```python
from build123d import *

# Parameters (mm, degrees)
SKETCH1_W                    = 110
SKETCH1_H                    = 200
SKETCH1_W_2                  = 70
SKETCH1_H_2                  = 120
BASE_FLANGE1_DEPTH           = 0.7366
EDGE_FLANGE1_STRIP_W         = 4.4196
EDGE_FLANGE1_STRIP_H         = 0.7366
EDGE_FLANGE1_STRIP_CUT_DEPTH = 200
EDGE_FLANGE1_DEPTH           = 200
EDGE_FLANGE2_STRIP_W         = 4.4196
EDGE_FLANGE2_STRIP_H         = 0.7366
EDGE_FLANGE2_STRIP_CUT_DEPTH = 200
EDGE_FLANGE2_DEPTH           = 200
EDGE_FLANGE3_STRIP_W         = 4.4196
EDGE_FLANGE3_STRIP_H         = 0.7366
EDGE_FLANGE3_STRIP_CUT_DEPTH = 108.5268
EDGE_FLANGE3_DEPTH           = 108.5268
EDGE_FLANGE3_START           = 0.7366
EDGE_FLANGE3_FLAT_DEPTH      = 0.7366
EDGE_FLANGE4_STRIP_W         = 4.4196
EDGE_FLANGE4_STRIP_H         = 0.7366
EDGE_FLANGE4_STRIP_CUT_DEPTH = 108.5268
EDGE_FLANGE4_DEPTH           = 108.5268
EDGE_FLANGE4_START           = 0.7366
EDGE_FLANGE4_FLAT_DEPTH      = 0.7366
CUT_EXTRUDE2_DEPTH           = 289.797370967
CUT_EXTRUDE3_START           = -0.7366
CUT_EXTRUDE3_DEPTH           = 0.7366
CUT_EXTRUDE6_DEPTH           = 800.082459726
CUT_EXTRUDE6_DEPTH_BACK      = 800.082459726
SKETCH53_R                   = 2.2
SKETCH53_R_2                 = 2.199999998
CUT_EXTRUDE7_DEPTH           = 10


# Read off the part's stored shape, not the designer's step: Cut-Extrude3
# Sheet-metal steps are written as plain solids
with BuildPart() as part:
    # Sketch1 → Base-Flange1 (new body)
    with BuildSketch(Plane(origin=(0, 0, 0), x_dir=(1, 0, 0), z_dir=(0, 1, 0))):
        Rectangle(SKETCH1_W, SKETCH1_H)
        Rectangle(SKETCH1_W_2, SKETCH1_H_2, mode=Mode.SUBTRACT)
    extrude(amount=-BASE_FLANGE1_DEPTH)

    # Edge-Flange1 strip (across the edge) → Edge-Flange1 strip cut (cut)
    with BuildSketch(Plane(origin=(-55, 0, -100), x_dir=(1, 0, 0), z_dir=(0, 0, 1))):
        with Locations((-1.4732, -0.3683)):
            Rectangle(EDGE_FLANGE1_STRIP_W, EDGE_FLANGE1_STRIP_H)
    extrude(amount=EDGE_FLANGE1_STRIP_CUT_DEPTH, mode=Mode.SUBTRACT)

    # Edge-Flange1 section (across the edge) → Edge-Flange1 (add)
    with BuildSketch(Plane(origin=(-55, 0, -100), x_dir=(1, 0, 0), z_dir=(0, 0, 1))):
        with BuildLine():
            Line((-0.7366, 0.7366), (-0.7366, 199.2634))
            Line((-0.7366, 199.2634), (0, 199.2634))
            Line((0, 199.2634), (0, 0.7366))
            ThreePointArc((0, 0.7366), (0.215745145, 0.215745145), (0.7366, 0))
            Line((0.7366, 0), (0.7366, -0.7366))
            ThreePointArc((0.7366, -0.7366), (-0.30510971, -0.30510971), (-0.7366, 0.7366))
        make_face()
    extrude(amount=EDGE_FLANGE1_DEPTH)

    # Edge-Flange2 strip (across the edge) → Edge-Flange2 strip cut (cut)
    with BuildSketch(Plane(origin=(55, 0, 100), x_dir=(-1, 0, 0), z_dir=(0, 0, -1))):
        with Locations((-1.4732, -0.3683)):
            Rectangle(EDGE_FLANGE2_STRIP_W, EDGE_FLANGE2_STRIP_H)
    extrude(amount=EDGE_FLANGE2_STRIP_CUT_DEPTH, mode=Mode.SUBTRACT)

    # Edge-Flange2 section (across the edge) → Edge-Flange2 (add)
    with BuildSketch(Plane(origin=(55, 0, 100), x_dir=(-1, 0, 0), z_dir=(0, 0, -1))):
        with BuildLine():
            Line((-0.7366, 0.7366), (-0.7366, 99.2634))
            Line((-0.7366, 99.2634), (0, 99.2634))
            Line((0, 99.2634), (0, 0.7366))
            ThreePointArc((0, 0.7366), (0.215745145, 0.215745145), (0.7366, 0))
            Line((0.7366, 0), (0.7366, -0.7366))
            ThreePointArc((0.7366, -0.7366), (-0.30510971, -0.30510971), (-0.7366, 0.7366))
        make_face()
    extrude(amount=EDGE_FLANGE2_DEPTH)

    # Edge-Flange3 strip (across the edge) → Edge-Flange3 strip cut (cut)
    with BuildSketch(Plane(origin=(54.2634, 0, -100), x_dir=(0, 0, 1), z_dir=(-1, 0, 0))):
        with Locations((-1.4732, -0.3683)):
            Rectangle(EDGE_FLANGE3_STRIP_W, EDGE_FLANGE3_STRIP_H)
    extrude(amount=EDGE_FLANGE3_STRIP_CUT_DEPTH, mode=Mode.SUBTRACT)

    # Edge-Flange3 bend section (across the edge) → Edge-Flange3 (add)
    with BuildSketch(Plane(origin=(54.2634, 0, -100), x_dir=(0, 0, 1), z_dir=(-1, 0, 0))):
        with BuildLine():
            Line((-0.7366, 0.7366), (0, 0.7366))
            ThreePointArc((0, 0.7366), (0.215745145, 0.215745145), (0.7366, 0))
            Line((0.7366, 0), (0.7366, -0.7366))
            ThreePointArc((0.7366, -0.7366), (-0.30510971, -0.30510971), (-0.7366, 0.7366))
        make_face()
    extrude(amount=EDGE_FLANGE3_DEPTH)

    # Edge-Flange3 profile (on flange) → Edge-Flange3 flat (add)
    with BuildSketch(Plane(origin=(0, 0, -100), x_dir=(-1, 0, 0), z_dir=(0, 0, -1)).offset(EDGE_FLANGE3_START)):
        Polygon((-54.2634, 115), (-54.2634, 0.7366), (54.2634, 0.7366), (54.2634, 199.2634), align=None)
    extrude(amount=-EDGE_FLANGE3_FLAT_DEPTH)

    # Edge-Flange4 strip (across the edge) → Edge-Flange4 strip cut (cut)
    with BuildSketch(Plane(origin=(-54.2634, 0, 100), x_dir=(0, 0, -1), z_dir=(1, 0, 0))):
        with Locations((-1.4732, -0.3683)):
            Rectangle(EDGE_FLANGE4_STRIP_W, EDGE_FLANGE4_STRIP_H)
    extrude(amount=EDGE_FLANGE4_STRIP_CUT_DEPTH, mode=Mode.SUBTRACT)

    # Edge-Flange4 bend section (across the edge) → Edge-Flange4 (add)
    with BuildSketch(Plane(origin=(-54.2634, 0, 100), x_dir=(0, 0, -1), z_dir=(1, 0, 0))):
        with BuildLine():
            Line((-0.7366, 0.7366), (0, 0.7366))
            ThreePointArc((0, 0.7366), (0.215745145, 0.215745145), (0.7366, 0))
            Line((0.7366, 0), (0.7366, -0.7366))
            ThreePointArc((0.7366, -0.7366), (-0.30510971, -0.30510971), (-0.7366, 0.7366))
        make_face()
    extrude(amount=EDGE_FLANGE4_DEPTH)

    # Edge-Flange4 profile (on flange) → Edge-Flange4 flat (add)
    with BuildSketch(Plane.XY.offset(100).offset(EDGE_FLANGE4_START)):
        Polygon((-54.2634, 199.2634), (-54.2634, 0.7366), (54.2634, 0.7366), (54.2634, 115), align=None)
    extrude(amount=-EDGE_FLANGE4_FLAT_DEPTH)

    # Sketch24 → Cut-Extrude2 (cut, through all)
    with BuildSketch(Plane(origin=(0, 0, -100.7366), x_dir=(-1, 0, 0), z_dir=(0, 0, -1))):
        Polygon((-28.519875042, 107.808063094), (31.460124178, 107.808063094), (31.460124178, 158.533542729), align=None)
        Polygon((-28.150641863, 10.732953924), (31.829357358, 10.732953924), (31.829357358, 61.45843356), align=None)
        Polygon((31.713150602, 88.173102361), (-28.636081798, 88.173102361), (-28.636081798, 37.135359798), align=None)
    extrude(amount=-CUT_EXTRUDE2_DEPTH, mode=Mode.SUBTRACT)

    # Cut-Extrude3 outline → Cut-Extrude3 (cut)
    with BuildSketch(Plane(origin=(55.7366, 0, 0), x_dir=(0, 0, -1), z_dir=(1, 0, 0)).offset(CUT_EXTRUDE3_START)):
        with BuildLine():
            Line((-87.713422796, 42.053472661), (-6.797155753, 39.040000774))
            add(Edge.make_bspline(
                [(-6.797155753, 39.040000774), (-87.713422796, 42.053472661), (67.110125935, 80.068334048), (60.312641059, 39.424036929), (22.052524279, 39.424036929)],
                knots=[0, 0, 0, 0, 0, 1, 1, 1, 1, 1], degree=4))
            Line((22.052524279, 39.424036929), (60.312641059, 39.424036929))
            ThreePointArc((60.312641059, 39.424036929), (80.917037974, 56.86865569), (67.110125935, 80.068334048))
            Line((67.110125935, 80.068334048), (-87.713422796, 42.053472661))
        make_face()
    extrude(amount=CUT_EXTRUDE3_DEPTH, mode=Mode.SUBTRACT)

    # Sketch53 → Cut-Extrude6 (cut, two sides: drawn at the far end of the back side and taken through both)
    with BuildSketch(Plane(origin=(344.115063699, 0, 561.793038506), x_dir=(-1, 0, 0), z_dir=(0, 1, 0)).offset(-CUT_EXTRUDE6_DEPTH_BACK)):
        with Locations(Location((392.463649434, -480.956438506, 0), (0, 0, 90))):
            Circle(SKETCH53_R)
        with Locations(Location((392.463649434, -465.956438506, 0), (0, 0, 90))):
            Circle(SKETCH53_R)
        with Locations(Location((362.463649434, -473.456438506, 0), (0, 0, 90))):
            Circle(SKETCH53_R)
        with Locations(Location((292.463649434, -480.956438506, 0), (0, 0, 90))):
            Circle(SKETCH53_R)
        with Locations(Location((292.463649434, -465.956438506, 0), (0, 0, 90))):
            Circle(SKETCH53_R)
        with Locations(Location((322.463649434, -473.456438506, 0), (0, 0, 90))):
            Circle(SKETCH53_R)
        with Locations(Location((294.03158687, -636.983238506, 0), (0, 0, 90))):
            Circle(SKETCH53_R_2)
        with Locations(Location((324.69158687, -646.983238506, 0), (0, 0, 90))):
            Circle(SKETCH53_R_2)
        with Locations(Location((346.36158687, -636.983238506, 0), (0, 0, 90))):
            Circle(SKETCH53_R_2)
        with Locations(Location((368.028253537, -646.983238506, 0), (0, 0, 90))):
            Circle(SKETCH53_R_2)
        with Locations(Location((389.694920203, -636.983238506, 0), (0, 0, 90))):
            Circle(SKETCH53_R_2)
    extrude(amount=CUT_EXTRUDE6_DEPTH + CUT_EXTRUDE6_DEPTH_BACK, mode=Mode.SUBTRACT)

    # Sketch54 → Cut-Extrude7 (cut)
    with BuildSketch(Plane.ZY.offset(55.7366)):
        Polygon((-37.376001553, 179.2634), (5.247996894, 179.2634), (80, 105.199675962), (80, 62.968137981), align=None)
        Polygon((-80, 179.2634), (-80, 137.031862019), (37.376001553, 20.7366), (80, 20.7366), align=None)
        Polygon((-47.87199534, 20.7366), (-5.247996894, 20.7366), (-80, 94.800324038), (-80, 52.568786057), align=None)
        Polygon((80, 179.2634), (80, 147.431213943), (47.87199534, 179.2634), align=None)
    extrude(amount=-CUT_EXTRUDE7_DEPTH, mode=Mode.SUBTRACT)


solid = part.part
```
For this review, take the finished solid that the model builds, in its own axes (mm). A direction names the side the tool comes from. Coordinates: 2 decimals unless noted, no trailing zeros. Order: outer loops, then holes, each group sorted by start corner. A loop starts at its lowest first (then second) coordinate and runs counter-clockwise, first axis right, second up. Notation, with made-up numbers: (67.25, 60) -> (93.25, 60) arc R6 cw to (93.25, 65) -> close; hole circle Ø7 at (13.25, 21.25). An arc over 180 degrees is marked (long way). Answer as CSV lines item,"result".
Q1. We need section B-B (z = -70). State the section outline as (x, y) points.
Model answer:
outline,"(-55.74, 0.74) arc R1.47 ccw to (-54.26, -0.74) -> (54.26, -0.74) arc R1.47 ccw to (55.74, 0.74) -> (55.74, 41.81) -> (55, 41.81) -> (55, 0.74) arc R0.74 cw to (54.26, 0) -> (-54.26, 0) arc R0.74 cw to (-55, 0.74) -> (-55, 42.66) -> (-55.74, 42.66) -> close; (-55.74, 84.89) -> (-55, 84.89) -> (-55, 127.12) -> (-55.74, 127.12) -> close; (-55.74, 169.36) -> (-55, 169.36) -> (-55, 199.26) -> (-55.74, 199.26) -> close; (55, 78.82) -> (55.74, 78.82) -> (55.74, 99.26) -> (55, 99.26) -> close"
Q2. Clearance check with flat-ended pins moving along their axes: pin 1 Ø10 at (x, z) = (-4, 63) entering from +Y; pin 2 Ø0.6 at (x, z) = (-12, 100.5) entering from +Y; pin 3 Ø0.7 at (y, z) = (51, -100.5) entering from +X. State where each tip first meets the part, or that it passes through.
Model answer:
pin 1,"stops at y = 0"
pin 2,"stops at y = 166.68"
pin 3,"stops at x = 54.26"
Q3. For faces 4 (the face through (-55.373, 163.124, 64.161)), 5 (the face through (-55, 123, -1)), 6 (the face through (1, 101, -100)), 7 (the face through (-55.373, 36.876, -64.161)), list the 3-axis set-ups (+Z, -Z, +X, -X, +Y, -Y) from which the entire face can be reached by the end or side of a thin tool; tool diameter is ignored.
Model answer:
face 4,"+X, -X"
face 5,"+Z, -Z, +Y"
face 6,"+Y"
face 7,"-X"
Q4. Draft analysis for pull direction Y (two halves, no side actions). For faces 1 (the face through (-37, -0.737, -1)), 2 (the face through (-55.37, 57.25, -42.1)), 3 (the face through (55.737, 49, 1)), state which applies: released by +Y, released by -Y, zero draft, split by the parting line, or undercut.
Model answer:
face 1,"released by -Y"
face 2,"undercut"
face 3,"zero draft"
Q5. We need section D-D (y = 187.5). State the section outline as (x, z) points.
Model answer:
outline,"(-55.74, -100) -> (-55, -100) -> (-55, 100) -> (-55.74, 100) -> close; (-54.26, -100.74) -> (-39.11, -100.74) -> (-39.11, -100) -> (-54.26, -100) -> close; (-54.26, 100) -> (-39.11, 100) -> (-39.11, 100.74) -> (-54.26, 100.74) -> close"
Q6. We need section A-A (y = 120). State the section outline as (x, z) points.
Model answer:
outline,"(-55.74, -100) -> (-55, -100) -> (-55, -62.81) -> (-55.74, -62.81) -> close; (-55.74, -20.19) -> (-55, -20.19) -> (-55, 22.44) -> (-55.74, 22.44) -> close; (-55.74, 65.06) -> (-55, 65.06) -> (-55, 100) -> (-55.74, 100) -> close; (-54.26, -100.74) -> (-31.46, -100.74) -> (-31.46, -100) -> (-54.26, -100) -> close; (-54.26, 100) -> (-31.46, 100) -> (-31.46, 100.74) -> (-54.26, 100.74) -> close; (14.1, -100.74) -> (47.82, -100.74) -> (47.82, -100) -> (14.1, -100) -> close; (14.1, 100) -> (47.82, 100) -> (47.82, 100.74) -> (14.1, 100.74) -> close"
Q7. Wall thickness on line 1 along Z through (x, y) = (10.5, 28.5); line 2 along X through (y, z) = (17, -88.5); line 3 along X through (y, z) = (128.5, -18.5): over which ranges is each line inside the solid? List them lowest first. Write a range as [from, to].
Model answer:
line 1,"z = [-100.74, -100], [100, 100.74]"
line 2,"x = [-55.74, -55], [55, 55.74]"
line 3,"x = [-55.74, -55]"
Q8. We need section C-C (y = 24.5). Count the separate pieces of the cut face and the enclosed holes in it, plus the area to 3 significant figures.
Model answer:
separate pieces,"8"
enclosed holes,"0"
area,"327 mm2"
